The model under review builds one solid part; all positions refer to its coordinate system, in mm. A direction names the side the tool comes from. Coordinates: 2 decimals unless noted, no trailing zeros. Order: outer loops, then holes, each group sorted by start corner. A loop starts at its lowest first (then second) coordinate and runs counter-clockwise, first axis right, second up. Notation, with made-up numbers: M -27,-19 L 26,-19 A13 ccw 26,-13 Z; hole C 86.25,50 d11. An arc over 180 degrees is marked long. Answer as CSV lines item,"result". Start each with the question number.
Q1. Machinability: for faces 1 (the face through (26, 11, 13)), 2 (the face through (-17.675, -21.199, 6.676)), 3 (the face through (9.257, 33.6, 0.26)), which of the approach directions +Z, -Z, +X, -X, +Y, -Y give a long, thin tool a straight path to every point of the face, cutting with its end or side? Answer none if there is none.
Q2. Wall thickness on L1, parallel to Z at x = -13.5, y = 0 (3 decimals); L2, parallel to Z at x = 12, y = 0 (3 decimals); L3, parallel to Y at x = -19, z = -16.5: over which ranges is each line inside the solid? List them lowest first. Write a range as [from, to].
Q3. For P1, Ø9.5, axis at x = 15.16, z = 0, coming from the +Y side; P2, Ø12, axis at x = -4, z = 11.5, coming from the +Y side; P3, Ø1, axis at x = 9, y = 11, coming from the -Z side, all flat-tipped, find the tip position at first contact; note any pin that passes through.
Q4. Consider section B-B on z = 0. Write out the cut boundary in (x, y) (3 decimals), and give its area (3 significant figures).
Q5. Consider section C-C on x = -10.5. Write out the cut boundary in (y, z) (3 decimals), and give its area (3 significant figures).
Q6. Consider section D-D on z = -13.5. Write out the cut boundary in (x, y).
Q7. Consider section A-A on y = 0. Write out the cut boundary in (x, z) (3 decimals), and give its area (3 significant figures).
Q8. The part is to be moulded in two halves that separate along Z. For faces 4 (the face through (0, -28, 43)), 5 (the face through (-5, -10, -15)), 6 (the face through (-14.79, 11.056, -49.787)), 7 (the face through (10.72, -12.6, -9.66)), say which applies: +Z half, -Z half, draft (parallel to the pull), parting line (faces both ways), or undercut.
from build123d import *

# Parameters (mm, degrees)
F0_R      = 53
F1_DEPTH  = 26
F2_R      = 51
F3_DEPTH  = 30
F6_R      = 22.225
F7_DEPTH  = 25
F4_R      = 15.875
F8_DEPTH  = 31
F7_FACE_R = 22.225
F9_DEPTH  = 25
F10_R     = 22.225
F11_DEPTH = 25
F12_R     = 5.904872
F13_DEPTH = 57


with BuildPart() as f1:
    # F0 (on Right) → F1 (new body)
    with BuildSketch(Plane.YZ):
        Circle(F0_R)
    extrude(amount=F1_DEPTH)

    # F2 (on face) → F3 (join)
    with BuildSketch(Plane(origin=(0, 0, 0), x_dir=(0, -1, 0), z_dir=(-1, 0, 0))):
        Circle(F2_R)
    extrude(amount=F3_DEPTH)

    # F6 (on face) → F7 (join)
    with BuildSketch(Plane(origin=(-30, 0, 0), x_dir=(0, -1, 0), z_dir=(-1, 0, 0))):
        Circle(F6_R)
    extrude(amount=F7_DEPTH)

    # F4 (on face) → F8 (cut)
    with BuildSketch(Plane.YZ.offset(26)):
        Circle(F4_R)
    extrude(amount=-F8_DEPTH, mode=Mode.SUBTRACT)

    # F7_face (on face) → F9 (cut)
    with BuildSketch(Plane(origin=(-55, 0, 0), x_dir=(0, -1, 0), z_dir=(-1, 0, 0))):
        Circle(F7_FACE_R)
    extrude(amount=-F9_DEPTH, mode=Mode.SUBTRACT)

    # F10 (on face) → F11 (cut)
    with BuildSketch(Plane(origin=(-30, 0, 0), x_dir=(0, -1, 0), z_dir=(-1, 0, 0))):
        Circle(F10_R)
    extrude(amount=-F11_DEPTH, mode=Mode.SUBTRACT)

    # F12 (on Front) → F13 (cut)
    with BuildSketch(Plane.XZ):
        with Locations((15.155762, 0)):
            Circle(F12_R)
    extrude(amount=-F13_DEPTH, mode=Mode.SUBTRACT)


solid = f1.part
Evaluation:
1,face 1,"+Z, -Z, +X, +Y, -Y"
1,face 2,"-X"
1,face 3,"+Y"
2,L1,"z = [-51, -22.225], [22.225, 51]"
2,L2,"z = [-53, -15.875], [15.875, 53]"
2,L3,"y = [-48.26, -14.89], [14.89, 48.26]"
3,P1,"stops at y = -15.15"
3,P2,"stops at y = 52.53"
3,P3,"stops at z = -51.95"
4,outline,"M -30,-51 L 0,-51 L 0,-53 L 26,-53 L 26,-15.875 L -5,-15.875 L -5,-22.225 L -30,-22.225 Z; M -30,22.225 L -5,22.225 L -5,15.875 L 9.251,15.875 L 9.251,53 L 0,53 L 0,51 L -30,51 Z; M 21.061,15.875 L 26,15.875 L 26,53 L 21.061,53 Z"
4,area,"3,280 mm²"
5,outline,"C 0,0 d102; hole C 0,0 d44.45"
5,area,"6,620 mm²"
6,outline,"M -30,-49.18 L 0,-49.18 L 0,-51.25 L 26,-51.25 L 26,-8.35 L -5,-8.35 L -5,-17.66 L -30,-17.66 Z; M -30,17.66 L -5,17.66 L -5,8.35 L 26,8.35 L 26,51.25 L 0,51.25 L 0,49.18 L -30,49.18 Z"
7,outline,"M -30,-51 L 0,-51 L 0,-53 L 26,-53 L 26,-15.875 L -5,-15.875 L -5,-22.225 L -30,-22.225 Z; M -30,22.225 L -5,22.225 L -5,15.875 L 26,15.875 L 26,53 L 0,53 L 0,51 L -30,51 Z"
7,area,"3,720 mm²"
8,face 4,"draft"
8,face 5,"undercut"
8,face 6,"parting line"
8,face 7,"undercut"
